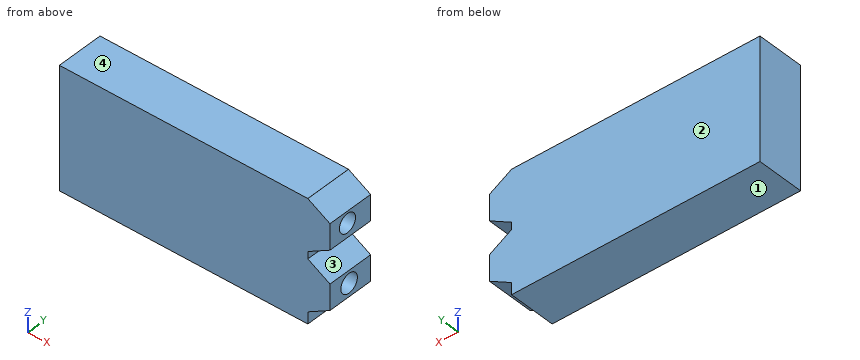
```python
from build123d import *

# Parameters (mm, degrees)
F0_W     = 42.183492
F0_H     = 20.596634
F2_DEPTH = 8
F3_DEPTH = 8
F4_R     = 1.624086
F5_DEPTH = 10
F6_R     = 1.584356
F7_DEPTH = 10


with BuildPart() as f2:
    # F0 (on Front) → F2 (new body)
    with BuildSketch(Plane.XZ):
        with Locations((-21.091746, 19.012278)):
            Rectangle(F0_W, F0_H)
    extrude(amount=F2_DEPTH)

    # F1 (on face) → F3 (join)
    with BuildSketch(Plane.XZ):
        Polygon((-3.762846, 27.126093), (-3.762846, 22.781133), (0, 20.608653), (3.762846, 22.781133), (3.762846, 27.126093), (0, 29.298573), align=None)
        Polygon((3.762846, 12.878906), (3.762846, 17.223866), (0, 19.396346), (-3.762846, 17.223866), (-3.762846, 12.878906), (0, 10.706426), align=None)
    extrude(amount=F3_DEPTH)

    # F4 (on face) → F5 (cut)
    with BuildSketch(Plane.YZ.offset(3.762846)):
        with Locations((-4.233076, 15.095317)):
            Circle(F4_R)
    extrude(amount=-F5_DEPTH, mode=Mode.SUBTRACT)

    # F6 (on face) → F7 (cut)
    with BuildSketch(Plane.YZ.offset(3.762846)):
        with Locations((-4.555025, 25.151657)):
            Circle(F6_R)
    extrude(amount=-F7_DEPTH, mode=Mode.SUBTRACT)


solid = f2.part
```
The listing builds one solid part. Answer for the finished solid, in the listing's coordinates (mm). Face numbers are marked on the shaded views. Round coordinates to 2 decimals unless told otherwise and drop trailing zeros. Loops run counter-clockwise (first coordinate to the right, second up) from the corner with the lowest first, then second, coordinate; pieces in that order, holes last.
1) A cutting plane is placed at D-D on z = 15.75. Determine the outline of the cut face in (x, y).
Outcome:
outline: (-42.18, -8) - (3.76, -8) - (3.76, -5.72) - (-6.24, -5.72) - (-6.24, -2.75) - (3.76, -2.75) - (3.76, 0) - (-42.18, 0) - close
2) Consider line 1 (Z direction, x = 2.5, y = -4.5); line 2 (X direction, y = -7.5, z = 10); line 3 (Y direction, x = -1, z = 15.5). Determine where each line is inside the solid, lowest interval first.
Outcome:
line 1: z = 12.15 to 13.49, 16.7 to 17.95, 22.05 to 23.57, 26.74 to 27.86
line 2: x = -42.18 to 0
line 3: y = -8 to -5.81, -2.66 to 0
3) For a pull along Z with two mould halves and no side action, classify the marked faces 1, 2, 3 and 4 as released by +Z, released by -Z, zero draft, split by the parting line, or undercut.
Outcome:
face 1: released by -Z
face 2: zero draft
face 3: undercut
face 4: released by +Z
4) A cutting plane is placed at B-B on z = 10.25. Determine the outline of the cut face in (x, y).
Outcome:
outline: (-42.18, -8) - (0, -8) - (0, 0) - (-42.18, 0) - close
5) Given P1, Ø1.6, axis at y = -5, z = 25, coming from the +X side; P2, Ø0.6, axis at y = -2, z = 9, coming from the +X side, each flat-ended and moving along its own axis, determine where each tip first touches the part or whether it passes through.
Outcome:
P1: stops at x = -6.24
P2: stops at x = 0
